Here's the drawing with two shaded views (mm, measured from the low corner). I have some questions. A direction names the side the tool comes from. Give positions to 0.01 mm unless a question says otherwise; leave off trailing zeros. Write each loop counter-clockwise with the first axis right and the second up, starting at its lowest first coordinate (ties: lowest second). Pieces come first, ordered by that corner, then holes. Notation, with made-up numbers: (59, 40.25) - (86, 40.25) arc R36 ccw to (86, 78.25) - close; hole circle Ø4 at (80, -37.75). An arc over 180 degrees is marked (long way). Answer as a JSON object with one key per item and string values. Group by question number.
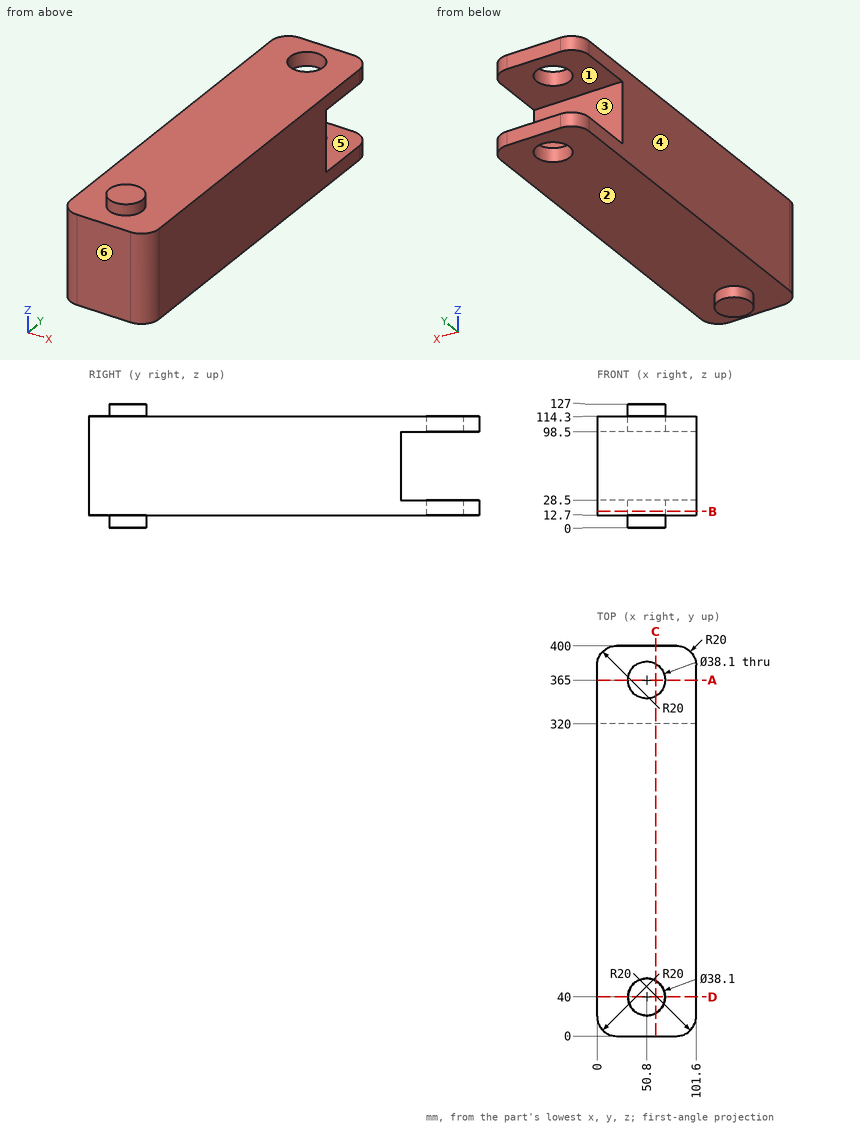
(1) Will these pins go through, and if not, where does the flat tip stop? P1, Ø1, axis at x = 17.5, z = 40, coming from the -Y side; P2, Ø1, axis at x = 61.5, y = 78.5, coming from the +Z side.
(2) I want a section at B-B, the plane z = 17. Please give me the cut outline in (x, y), and give its area (3 significant figures).
(3) I want a section at C-C, the plane x = 60. Please give me the cut outline in (y, z), and give its area (3 significant figures).
(4) I want a section at D-D, the plane y = 40. Please give me the cut outline in (x, z), and give its area (3 significant figures).
(5) I need wall thicknesses on L1, parallel to Z at x = 63, y = 347; L2, parallel to Y at x = 50.8, z = 19.5; L3, parallel to Z at x = 42.5, y = 159. Which ranges of each line are inside material? Lowest first, please.
(6) If we mould it in two halves opening along Z, with no side actions, what happens to the marked faces 1, 2, 3 and 4? For each: +Z half, -Z half, draft (parallel to the pull), parting line (faces both ways), or undercut.
(7) I want a section at A-A, the plane y = 365. Please give me the cut outline in (x, z), and give its area (3 significant figures).
(8) For the marked faces 5 and 6, which set-ups out of +Z, -Z, +X, -X, +Y, -Y let a thin tool reach every point of the face, with its end or its side?
Entries:
{
 "1": {"P1": "y = 0.1", "P2": "z = 114.3"},
 "2": {"outline": "(0, 20) arc R20 ccw to (20, 0) - (81.6, 0) arc R20 ccw to (101.6, 20) - (101.6, 380) arc R20 ccw to (81.6, 400) - (20, 400) arc R20 ccw to (0, 380) - close; hole circle Ø38.1 at (50.8, 365)", "area": "39,200 mm^2"},
 "3": {"outline": "(0, 12.7) - (23.32, 12.7) - (23.32, 0) - (56.68, 0) - (56.68, 12.7) - (348.32, 12.7) - (348.32, 28.5) - (320, 28.5) - (320, 98.5) - (348.32, 98.5) - (348.32, 114.3) - (56.68, 114.3) - (56.68, 127) - (23.32, 127) - (23.32, 114.3) - (0, 114.3) - close; (381.68, 12.7) - (400, 12.7) - (400, 28.5) - (381.68, 28.5) - close; (381.68, 98.5) - (400, 98.5) - (400, 114.3) - (381.68, 114.3) - close", "area": "34,800 mm^2"},
 "4": {"outline": "(0, 12.7) - (31.75, 12.7) - (31.75, 0) - (69.85, 0) - (69.85, 12.7) - (101.6, 12.7) - (101.6, 114.3) - (69.85, 114.3) - (69.85, 127) - (31.75, 127) - (31.75, 114.3) - (0, 114.3) - close", "area": "11,300 mm^2"},
 "5": {"L1": "12.7 to 28.5, 98.5 to 114.3", "L2": "0 to 345.95, 384.05 to 400", "L3": "12.7 to 114.3"},
 "6": {"face 1": "undercut", "face 2": "-Z half", "face 3": "undercut", "face 4": "draft"},
 "7": {"outline": "(0, 12.7) - (31.75, 12.7) - (31.75, 28.5) - (0, 28.5) - close; (0, 98.5) - (31.75, 98.5) - (31.75, 114.3) - (0, 114.3) - close; (69.85, 12.7) - (101.6, 12.7) - (101.6, 28.5) - (69.85, 28.5) - close; (69.85, 98.5) - (101.6, 98.5) - (101.6, 114.3) - (69.85, 114.3) - close", "area": "2,010 mm^2"},
 "8": {"face 5": "+X, -X, +Y", "face 6": "+Z, -Z, +X, -X, -Y"}
}
